Part model, mm, in its own coordinate system. A direction names the side the tool comes from. Round coordinates to 2 decimals unless told otherwise and drop trailing zeros. Loops run counter-clockwise (first coordinate to the right, second up) from the corner with the lowest first, then second, coordinate; pieces in that order, holes last. Notation, with made-up numbers: M 85,-26 L 113,-26 A18 ccw 113,-17 Z; hole C -36,48 d8. An arc over 180 degrees is marked long. Put each result on its own line as item: value. Start each with the question number.
```python
from build123d import *

# Parameters (mm, degrees)
SKETCH1_R           = 3.5
BOSS_EXTRUDE1_DEPTH = 5
SKETCH2_R           = 4
BOSS_EXTRUDE2_DEPTH = 5
SKETCH3_R           = 3.5
BOSS_EXTRUDE3_DEPTH = 35


with BuildPart() as part:
    # Sketch1 → Boss-Extrude1 (new body)
    with BuildSketch(Plane(origin=(0, 0, 0), x_dir=(1, 0, 0), z_dir=(0, 1, 0))):
        with Locations(Location((0, 0, 0), (0, 0, 270))):  # turned: the seam where the file's is
            Circle(SKETCH1_R)
    extrude(amount=BOSS_EXTRUDE1_DEPTH)

    # Sketch2 → Boss-Extrude2 (add)
    with BuildSketch(Plane(origin=(0, 5, 0), x_dir=(1, 0, 0), z_dir=(0, 1, 0))):
        with Locations(Location((0, 0, 0), (0, 0, 270))):  # turned: the seam where the file's is
            Circle(SKETCH2_R)
    extrude(amount=BOSS_EXTRUDE2_DEPTH)

    # Sketch3 → Boss-Extrude3 (add)
    with BuildSketch(Plane(origin=(0, 10, 0), x_dir=(1, 0, 0), z_dir=(0, 1, 0))):
        with Locations(Location((0, 0, 0), (0, 0, 270))):  # turned: the seam where the file's is
            Circle(SKETCH3_R)
    extrude(amount=BOSS_EXTRUDE3_DEPTH)


solid = part.part
```
1. Cut at C-C, the plane y = 19. Give the cut face in (x, z), and give its area (3 significant figures).
2. Cut at B-B, the plane z = 0. Give the cut face in (x, y), and give its area (3 significant figures).
3. Which spindle directions (+Z, -Z, +X, -X, +Y, -Y) get a long thin tool onto all of the face, cutting with end or side? Do faces 1 (the cylindrical face through (-3.417, 2.465, -0.759)), 2 (the cylindrical face through (-3.417, 27.255, -0.759)), 3 (the flat face through (0, 45, 0)). Say none if no direction does.
4. Drop flat-ended pins along their axis: pin 1 (3 mm diameter, centred on x = 1, y = 38.5, fed in from -Z); pin 2 (4 mm diameter, centred on y = 13, z = 1.5, fed in from +X); pin 3 (2 mm diameter, centred on y = 18, z = 3, fed in from -X). Give the stop position or say it passes through.
5. Wall check: L1, parallel to Z at x = 0.25, y = 26; L2, parallel to Y at x = 1.5, z = 3.25; L3, parallel to X at y = 11, z = -0.5. Give the ranges that are in metal, low to high.
6. Cut at A-A, the plane x = 0. Give the cut face in (y, z).
Results list:
1. outline: C 0,0 d7
1. area: 38.5 mm^2
2. outline: M -4,5 L -3.5,5 L -3.5,0 L 3.5,0 L 3.5,5 L 4,5 L 4,10 L 3.5,10 L 3.5,45 L -3.5,45 L -3.5,10 L -4,10 Z
2. area: 320 mm^2
3. face 1: -Y
3. face 2: +Y
3. face 3: +Z, -Z, +X, -X, +Y
4. pin 1: stops at z = -3.5
4. pin 2: stops at x = 3.5
4. pin 3: stops at x = -2.87
5. L1: z = -3.49 to 3.49
5. L2: y = 5 to 10
5. L3: x = -3.46 to 3.46
6. outline: M 0,-3.5 L 5,-3.5 L 5,-4 L 10,-4 L 10,-3.5 L 45,-3.5 L 45,3.5 L 10,3.5 L 10,4 L 5,4 L 5,3.5 L 0,3.5 Z
